Could you check a few things on this model? Use its own coordinates, in mm. Face numbers are marked on the shaded views. A direction names the side the tool comes from. Give positions to 0.01 mm unless a question says otherwise; leave off trailing zeros. Order: outer loops, then holes, each group sorted by start corner. A loop starts at its lowest first (then second) coordinate and runs counter-clockwise, first axis right, second up. Notation, with made-up numbers: M 18,-31 L 26,-31 A19 cw 26,-3 Z; hole C 0,-34.5 d10. An arc over 180 degrees is marked long. Use a Markdown table: item, result. Add a question column.
Item 1: I'm going to push flat-ended pins straight in: pin 1 Ø8 at (x, z) = (-6, 35) entering from +Y; pin 2 Ø3 at (y, z) = (5, 25) entering from -X. Where does each tip first touch, or does it pass through?
Item 2: Suppose I cut it at B-B on z = 20. Write out the boundary of the cut face in (x, y), plus the area to 3 significant figures.
Item 3: For the marked faces 1 and 2, which set-ups out of +Z, -Z, +X, -X, +Y, -Y let a thin tool reach every point of the face, with its end or its side?
Item 4: Suppose I cut it at C-C on y = 9. Write out the boundary of the cut face in (x, z).
Item 5: If I drill on L1, parallel to Z at x = -12, y = 0.55; L2, parallel to Z at x = -0.3, y = 9; L3, parallel to Y at x = -13, z = 24.5, over which ranges is the centre line in solid material (lowest first)? Write a range as from..to.
Item 6: Suppose I cut it at A-A on x = -12. Write out the boundary of the cut face in (y, z).
Item 7: Suppose I cut it at D-D on z = 30. Write out the boundary of the cut face in (x, y).
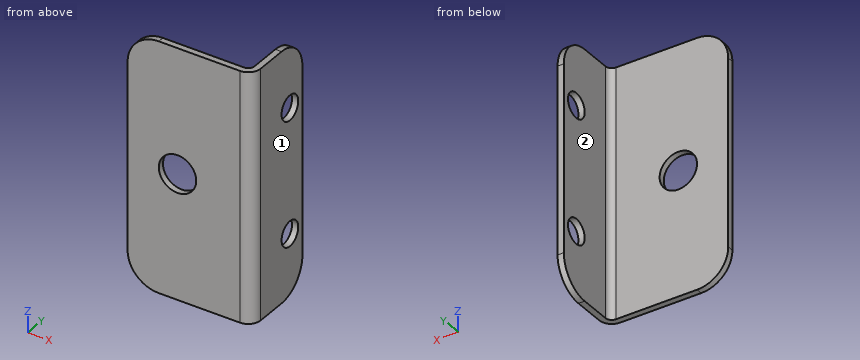
from build123d import *

# Parameters (mm, degrees)
BASE_FLANGE1_DEPTH      = 40
CUT_EXTRUDE1_DEPTH      = 47.054315759
CUT_EXTRUDE1_DEPTH_BACK = 47.054315759
SKETCH6_R               = 3
CUT_EXTRUDE2_DEPTH      = 46.880278988
CUT_EXTRUDE2_DEPTH_BACK = 46.880278988
SKETCH7_R               = 2
FILLET1_R               = 5


# Sheet-metal steps are written as plain solids
with BuildPart() as part:
    # Sketch1 → Base-Flange1 (new body)
    with BuildSketch(Plane.XY):
        with BuildLine():
            Line((0, 12), (0, 2))
            ThreePointArc((0, 2), (-0.585786438, 0.585786438), (-2, 0))
            Line((-2, 0), (-20, 0))
            Line((-20, 0), (-20, 1))
            Line((-20, 1), (-2, 1))
            ThreePointArc((-2, 1), (-1.292893219, 1.292893219), (-1, 2))
            Line((-1, 2), (-1, 12))
            Line((-1, 12), (0, 12))
        make_face()
    extrude(amount=BASE_FLANGE1_DEPTH)

    # Sketch6 → Cut-Extrude1 (cut, two sides: drawn at the far end of the back side and taken through both)
    with BuildSketch(Plane(origin=(0, 1, 0), x_dir=(1, 0, 0), z_dir=(0, 1, 0)).offset(-CUT_EXTRUDE1_DEPTH_BACK)):
        with Locations(Location((-12, -20, 0), (0, 0, 180))):
            Circle(SKETCH6_R)
    extrude(amount=CUT_EXTRUDE1_DEPTH + CUT_EXTRUDE1_DEPTH_BACK, mode=Mode.SUBTRACT)

    # Sketch7 → Cut-Extrude2 (cut, two sides: drawn at the far end of the back side and taken through both)
    with BuildSketch(Plane.ZY.offset(1).offset(-CUT_EXTRUDE2_DEPTH_BACK)):
        with Locations((10, 9)):
            Circle(SKETCH7_R)
        with Locations((30, 9)):
            Circle(SKETCH7_R)
    extrude(amount=CUT_EXTRUDE2_DEPTH + CUT_EXTRUDE2_DEPTH_BACK, mode=Mode.SUBTRACT)

    # Fillet1
    fillet1_edges = [part.edges().sort_by_distance(p)[0] for p in [
        (-0.5, 12, 40),
        (-0.5, 12, 0),
        (-20, 0.5, 40),
        (-20, 0.5, 0),
    ]]
    fillet(fillet1_edges, radius=FILLET1_R)


solid = part.part
Findings below:
| question | item | result |
|---|---|---|
| 1 | pin 1 | stops at y = 1 |
| 1 | pin 2 | stops at x = -1 |
| 2 | outline | M -20,0 L -15,0 L -15,1 L -20,1 Z; M -9,0 L -2,0 A2 ccw 0,2 L 0,12 L -1,12 L -1,2 A1 cw -2,1 L -9,1 Z |
| 2 | area | 24.4 mm^2 |
| 3 | face 1 | +Z, -Z, +X, +Y, -Y |
| 3 | face 2 | +Z, -Z, -X, +Y |
| 4 | outline | M -1,0.42 L 0,0.42 L 0,8 L -1,8 Z; M -1,12 L 0,12 L 0,28 L -1,28 Z; M -1,32 L 0,32 L 0,39.58 L -1,39.58 Z |
| 5 | L1 | z = 0..17, 23..40 |
| 5 | L2 | z = 0.42..8, 12..28, 32..39.58 |
| 5 | L3 | y = 0..1 |
| 6 | outline | M 0,0 L 1,0 L 1,17 L 0,17 Z; M 0,23 L 1,23 L 1,40 L 0,40 Z |
| 7 | outline | M -20,0 L -2,0 A2 ccw 0,2 L 0,7 L -1,7 L -1,2 A1 cw -2,1 L -20,1 Z; M -1,11 L 0,11 L 0,12 L -1,12 Z |
